Work out the finished part from the listing and answer in its coordinate system (mm). Face numbers are marked on the shaded views. A direction names the side the tool comes from. Coordinates: 2 decimals unless noted, no trailing zeros. Loops run counter-clockwise (first coordinate to the right, second up) from the corner with the lowest first, then second, coordinate; pieces in that order, holes last. Notation, with made-up numbers: (-25, 64) - (21, 64) arc R29 ccw to (21, 88) - close; hole circle Ø11 at (-13.5, -14). An arc over 180 degrees is marked (long way). Write each question's results on one line, items separated by ' | '. Start each with the question number.
1. A cutting plane is placed at A-A on y = 0. State how many separate pieces and enclosed holes the cut face has, then the cut area to 3 significant figures.
2. Each of these flat-tipped pins is pushed along its axis until it touches: P1, Ø4, axis at y = -20.5, z = -8.5, coming from the -X side; P2, Ø0.8, axis at y = 0.5, z = 0.5, coming from the +X side. Where does it stop, or does it pass through?
3. A cutting plane is placed at D-D on x = -21.25. Determine the outline of the cut face in (y, z).
4. Find the intervals of material crossed by line 1 along Z through (x, y) = (-1.5, 0); line 2 along Z through (x, y) = (-1.35, 4.85); line 3 along Z through (x, y) = (-2.5, 2.5), in increasing order. Write a range as [from, to].
5. Which of the six approach directions +Z, -Z, +X, -X, +Y, -Y give full straight-line access (tool end or side, diameter ignored) to the marked faces 1 and 2?
from build123d import *

# Parameters (mm, degrees)
F3_DEPTH = 6
F5_R     = 7
F5_R_2   = 2
F5_R_3   = 1.625392
F6_DEPTH = 2


with BuildPart() as f1:
    # F0 (on Front) → F1 (revolve)
    with BuildSketch(Plane.XZ):
        with BuildLine():
            Line((-2, 25), (-2, 8))
            ThreePointArc((-2, 8), (-2.87868, 5.87868), (-5, 5))
            Line((-5, 5), (-17, 5))
            Line((-17, 5), (-17, 3))
            Line((-17, 3), (-24, 3))
            Line((-24, 3), (-24, 0))
            Line((-24, 0), (-17, 0))
            Line((-17, 0), (-6, 0))
            Line((-6, 0), (-6, 1.6))
            Line((-6, 1.6), (0, 1.6))
            Line((0, 1.6), (0, 28))
            Line((0, 28), (0, 30))
            Line((0, 30), (-10, 30))
            Line((-10, 30), (-10, 28))
            Line((-10, 28), (-5, 28))
            ThreePointArc((-5, 28), (-2.87868, 27.12132), (-2, 25))
        make_face()
    revolve(axis=Axis((-36.628073, 0, 0), (1, 0, 0)))

    # F2 (on face) → F3 (join)
    with BuildSketch(Plane.YZ):
        with BuildLine():
            Line((1.249, -1), (-1.249, -1))
            ThreePointArc((-1.249, -1), (0, -1.6), (1.249, -1))
        make_face()
    extrude(amount=-F3_DEPTH)

    # F5 (on face) → F6 (cut)
    with BuildSketch(Plane(origin=(-2, 0, 0), x_dir=(0, -1, 0), z_dir=(-1, 0, 0))):
        with Locations((0, 17.75)):
            Circle(F5_R)
        with Locations((-15.371951, 8.875)):
            Circle(F5_R)
        with Locations((-15.371951, -8.875)):
            Circle(F5_R)
        with Locations((0, -17.75)):
            Circle(F5_R)
        with Locations((15.371951, -8.875)):
            Circle(F5_R)
        with Locations((15.371951, 8.875)):
            Circle(F5_R)
        with Locations((-11, 19.052559)):
            Circle(F5_R_2)
        with Locations((-4.85, 8.400446)):
            Circle(F5_R_3)
        with Locations((-22, 0)):
            Circle(F5_R_2)
        with Locations((-9.7, 0)):
            Circle(F5_R_3)
        with Locations((-11, -19.052559)):
            Circle(F5_R_2)
        with Locations((-4.85, -8.400446)):
            Circle(F5_R_3)
        with Locations((11, -19.052559)):
            Circle(F5_R_2)
        with Locations((4.85, -8.400446)):
            Circle(F5_R_3)
        with Locations((22, 0)):
            Circle(F5_R_2)
        with Locations((9.7, 0)):
            Circle(F5_R_3)
        with Locations((11, 19.052559)):
            Circle(F5_R_2)
        with Locations((4.85, 8.400446)):
            Circle(F5_R_3)
    extrude(amount=-F6_DEPTH, mode=Mode.SUBTRACT)


solid = f1.part
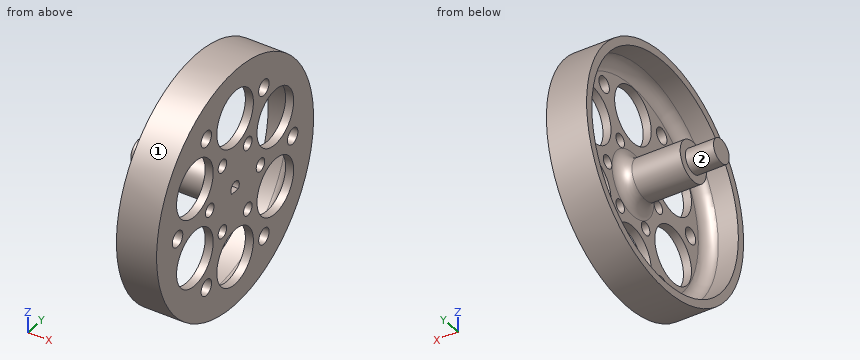
Values:
1) separate pieces: 3 | enclosed holes: 0 | area: 280 mm^2
2) P1: x = -2 | P2: x = -6
3) outline: circle Ø6 at (0, 0)
4) line 1: [-30, -24.75], [-10.75, -1], [1.6, 10.75], [24.75, 30] | line 2: [-29.61, -22.8], [-12.7, -10.03], [-6.78, 6.78], [10.03, 12.7], [22.8, 29.61] | line 3: [-29.9, -26.54], [-5.83, 5.83], [26.54, 29.9]
5) face 1: +X, -X | face 2: -X
